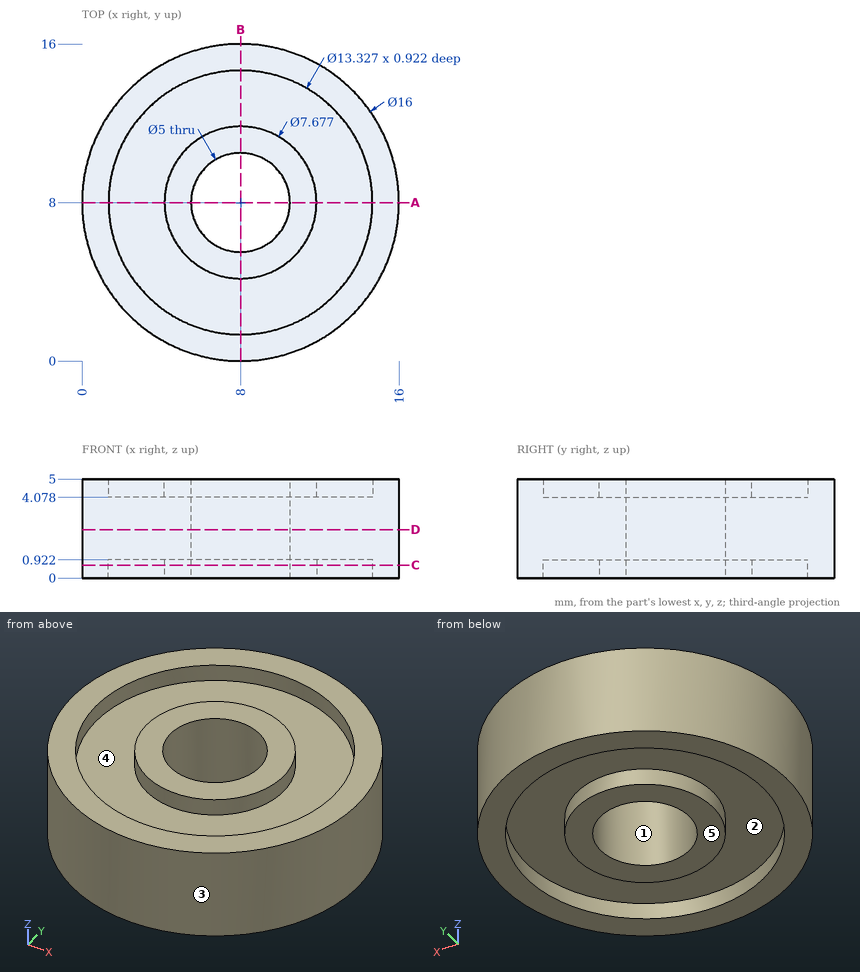
Study the drawing (mm; zero at the part's minimum x, y, z) and answer. A direction names the side the tool comes from. Coordinates: 2 decimals unless noted, no trailing zeros. Write each loop counter-clockwise with the first axis right and the second up, starting at its lowest first coordinate (ties: lowest second). Pieces come first, ordered by that corner, then holes.
Q1. Which of the six approach directions +Z, -Z, +X, -X, +Y, -Y give full straight-line access (tool end or side, diameter ignored) to the marked faces 1 and 2?
Q2. A cutting plane is placed at D-D, the plane z = 2.45. Give the vertices of the cut face in (x, y).
Q3. A cutting plane is placed at C-C, the plane z = 0.65. Give the vertices of the cut face in (x, y).
Q4. A cutting plane is placed at A-A, the plane y = 8. Give the vertices of the cut face in (x, z).
Q5. Each of these flat-tipped pins is pushed along its axis until it touches: pin 1 Ø1 at (x, z) = (13.5, 2.5) entering from -Y (1 decimal); pin 2 Ø4.5 at (x, y) = (8, 8) entering from +Z; pin 3 Ø3 at (y, z) = (13.5, 2) entering from +X. Where does it stop, or does it pass through?
Q6. Find the intervals of material crossed by line 1 (Y direction, x = 4.5, z = 4.2) (1 decimal); line 2 (Y direction, x = 8, z = 3.1); line 3 (X direction, y = 6.75, z = 4.25) (1 decimal), in increasing order.
Q7. Determine the mould class of the marked faces 3, 4 and 5 for opening direction Y: released by +Y, released by -Y, zero draft, split by the parting line, or undercut.
Findings below:
1. face 1: +Z, -Z
1. face 2: -Z
2. outline: circle Ø16 at (8, 8); hole circle Ø5 at (8, 8)
3. outline: circle Ø16 at (8, 8); circle Ø7.68 at (8, 8); hole circle Ø13.33 at (8, 8); hole circle Ø5 at (8, 8)
4. outline: (0, 0) - (1.34, 0) - (1.34, 0.92) - (4.16, 0.92) - (4.16, 0) - (5.5, 0) - (5.5, 5) - (4.16, 5) - (4.16, 4.08) - (1.34, 4.08) - (1.34, 5) - (0, 5) - close; (10.5, 0) - (11.84, 0) - (11.84, 0.92) - (14.66, 0.92) - (14.66, 0) - (16, 0) - (16, 5) - (14.66, 5) - (14.66, 4.08) - (11.84, 4.08) - (11.84, 5) - (10.5, 5) - close
5. pin 1: stops at y = 1.8
5. pin 2: passes through
5. pin 3: stops at x = 14.93
6. line 1: y = 0.8 to 2.3, 6.4 to 9.6, 13.7 to 15.2
6. line 2: y = 0 to 5.5, 10.5 to 16
6. line 3: x = 0.1 to 1.5, 4.4 to 5.8, 10.2 to 11.6, 14.5 to 15.9
7. face 3: split by the parting line
7. face 4: undercut
7. face 5: zero draft
